from build123d import *

# Parameters (mm, degrees)
F0_W     = 25.4
F0_H     = 25.4
F1_DEPTH = 50.8
F2_DEPTH = 25.4
F3_W     = 25.4
F3_H     = 25.4
F4_DEPTH = 25.4
F5_W     = 25.4
F5_H     = 25.4
F6_DEPTH = 25.4


with BuildPart() as f1:
    # F0 (on Front) → F1 (new body)
    with BuildSketch(Plane.XZ):
        with Locations((-31.858784, -1.663636)):
            Rectangle(F0_W, F0_H)
    extrude(amount=F1_DEPTH)

    # F0 (on Front) → F2 (join)
    with BuildSketch(Plane.XZ):
        with Locations((18.941216, -1.663636)):
            Rectangle(F0_W, F0_H)
        with Locations((-6.458784, -1.663636)):
            Rectangle(F0_W, F0_H)
    extrude(amount=F2_DEPTH)

    # F3 (on face) → F4 (join)
    with BuildSketch(Plane.XZ):
        with Locations((-6.458784, -1.663636)):
            Rectangle(F3_W, F3_H)
    extrude(amount=-F4_DEPTH)

    # F5 (on face) → F6 (join)
    with BuildSketch(Plane(origin=(0, 0, -14.363636), x_dir=(1, 0, 0), z_dir=(0, 0, -1))):
        with Locations((-6.458784, -12.7)):
            Rectangle(F5_W, F5_H)
    extrude(amount=F6_DEPTH)


solid = f1.part
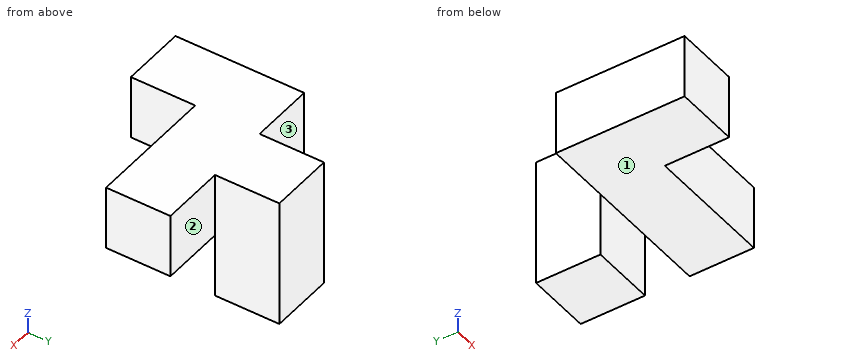
Design review of the part built by this model. Coordinates are the model's own, in mm. Face numbers are marked on the shaded views. A direction names the side the tool comes from. Round coordinates to 2 decimals unless told otherwise and drop trailing zeros. Write each loop counter-clockwise with the first axis right and the second up, starting at its lowest first coordinate (ties: lowest second). Pieces come first, ordered by that corner, then holes. Notation, with made-up numbers: (69.25, -28) -> (122.25, -28) arc R26 cw to (122.25, 8) -> close; hole circle Ø6 at (-11, 72). An arc over 180 degrees is marked (long way). One line per item, written item: value. Start each with the question number.
Q1. Add section A-A (z = -1). Give the boundary of the cut face in (x, y), then the cut area to 3 significant figures.
Q2. Add section B-B (x = 0.5). Give the boundary of the cut face in (y, z).
Q3. Add section D-D (z = -17). Give the boundary of the cut face in (x, y).
Q4. Tool access review of the marked faces 1, 2 and 3: name each direction out of +Z, -Z, +X, -X, +Y, -Y from which nothing blocks a thin tool from reaching the whole face with its end or side.
Q5. Add section C-C (y = -29.5). Give the boundary of the cut face in (x, z).
Q6. Insertion check: P1, Ø7.5, axis at x = 14, z = 4.5, coming from the -Y side; P2, Ø12.5, axis at x = -5.5, z = -32.5, coming from the -Y side; P3, Ø7.5, axis at y = 10, z = -23, coming from the +X side; P4, Ø20.5, axis at y = 9, z = -3.5, coming from the -X side. Each pin has a flat end and moves straight along its axis. Give the tip position at first contact, or say it passes through.
Q7. To check wall thickness, follow probe 1 along Z at (x, y) = (-28, -2); probe 2 along X at (y, z) = (18, -12.5); probe 3 along X at (y, z) = (-32, 7). State the ranges of each line that lie inside material, in increasing order.
Response:
1. outline: (-44.56, -50.8) -> (-19.16, -50.8) -> (-19.16, -25.4) -> (31.64, -25.4) -> (31.64, 0) -> (6.24, 0) -> (6.24, 25.4) -> (-19.16, 25.4) -> (-19.16, 0) -> (-44.56, 0) -> close
1. area: 3,230 mm^2
2. outline: (-25.4, -14.36) -> (0, -14.36) -> (0, -39.76) -> (25.4, -39.76) -> (25.4, 11.04) -> (-25.4, 11.04) -> close
3. outline: (-19.16, 0) -> (6.24, 0) -> (6.24, 25.4) -> (-19.16, 25.4) -> close
4. face 1: -Z, +X, -X, -Y
4. face 2: +Z, -Z, +X, +Y
4. face 3: +Z, -Z, -X, +Y
5. outline: (-44.56, -14.36) -> (-19.16, -14.36) -> (-19.16, 11.04) -> (-44.56, 11.04) -> close
6. P1: stops at y = -25.4
6. P2: stops at y = 0
6. P3: stops at x = 6.24
6. P4: stops at x = -44.56
7. probe 1: z = -14.36 to 11.04
7. probe 2: x = -19.16 to 6.24
7. probe 3: x = -44.56 to -19.16
